Can you work these out from the model? Positions are in its coordinate system, mm. Round coordinates to 2 decimals unless told otherwise and drop trailing zeros. Order: outer loops, then holes, each group sorted by start corner. A loop starts at its lowest first (then second) coordinate and runs counter-clockwise, first axis right, second up.
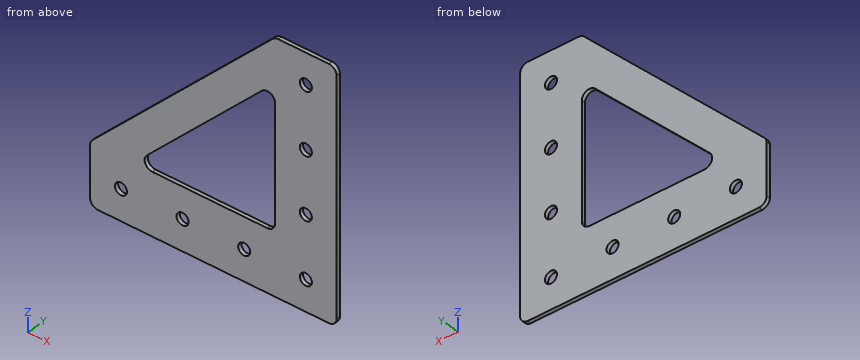
from build123d import *

# Parameters (mm, degrees)
BOSS_EXTRUDE1_DEPTH = 1.5875
SKETCH2_R           = 2.4892
CUT_EXTRUDE1_DEPTH  = 2.5875
LPATTERN1_COUNT     = 4
LPATTERN1_PITCH     = 25.4
LPATTERN1_COL_COUNT = 4
LPATTERN1_COL_PITCH = 25.4
FILLET1_R           = 3.175


with BuildPart() as part:
    # Sketch1 → Boss-Extrude1 (new body)
    with BuildSketch(Plane(origin=(0, 0, 0), x_dir=(1, 0, 0), z_dir=(0, 1, 0))):
        Polygon((0, 0), (-101.6, 0), (-101.6, -25.4), (-25.4, -101.6), (0, -101.6), align=None)
        Polygon((-25.4, -25.4), (-25.4, -83.639487758), (-83.639487758, -25.4), align=None, mode=Mode.SUBTRACT)
    extrude(amount=BOSS_EXTRUDE1_DEPTH)

    # Sketch2 → Cut-Extrude1 (cut, through all)
    with BuildSketch(Plane(origin=(0, 1.5875, 0), x_dir=(1, 0, 0), z_dir=(0, 1, 0))):
        with Locations((-12.7, -12.7)):
            Circle(SKETCH2_R)
    cut_extrude1 = extrude(amount=-CUT_EXTRUDE1_DEPTH, mode=Mode.SUBTRACT)

    # LPattern1: Cut-Extrude1 ×4
    with Locations(*[(0, 0, i * LPATTERN1_PITCH) for i in range(1, LPATTERN1_COUNT)]):
        add(cut_extrude1, mode=Mode.SUBTRACT)

    # LPattern1 col: Cut-Extrude1 ×4
    with Locations(*[(-i * LPATTERN1_COL_PITCH, 0, 0) for i in range(1, LPATTERN1_COL_COUNT)]):
        add(cut_extrude1, mode=Mode.SUBTRACT)

    # Fillet1
    fillet1_edges = [part.edges().sort_by_distance(p)[0] for p in [
        (-83.639487758, 0.79375, 25.4),
        (-25.4, 0.79375, 83.639487758),
        (-25.4, 0.79375, 25.4),
        (0, 0.79375, 101.6),
        (-25.4, 0.79375, 101.6),
        (-101.6, 0.79375, 25.4),
        (-101.6, 0.79375, 0),
        (0, 0.79375, 0),
    ]]
    fillet(fillet1_edges, radius=FILLET1_R)


solid = part.part
(1) I want a section at A-A, the plane z = 88.9. List the corners of the cut face in (x, y) for me.
(2) I want a section at C-C, the plane y = 0.7. Give the number of separate pieces and of enclosed holes in the cut face, plus the area to 3 significant figures.
(3) Please list where these lines run through material, in increasing order: probe 1 along X at (y, z) = (0.3, 12.7); probe 2 along Z at (x, y) = (-12.7, 0.55); probe 3 along X at (y, z) = (0.85, 38).
(4) I want a section at D-D, the plane x = -38.1. List the corners of the cut face in (y, z) for me.
(5) I want a section at B-B, the plane x = -12. List the corners of the cut face in (y, z) for me, plus the area to 3 significant figures.
(6) I'm going to push flat-ended pins straight in: pin 1 Ø4.5 at (x, z) = (-38.1, 12.7) entering from +Y; pin 2 Ø0.5 at (x, y) = (-48.5, 0.5) entering from +Z. Where does each tip first touch, or does it pass through?
Ans:
1. outline: (-38.1, 0) - (-15.19, 0) - (-15.19, 1.59) - (-38.1, 1.59) - close; (-10.21, 0) - (0, 0) - (0, 1.59) - (-10.21, 1.59) - close
2. separate pieces: 1
2. enclosed holes: 8
2. area: 5,610 mm2
3. probe 1: x = -101.6 to -91.39, -86.41 to -65.99, -61.01 to -40.59, -35.61 to -15.19, -10.21 to 0
3. probe 2: z = 0 to 10.21, 15.19 to 35.61, 40.59 to 61.01, 65.99 to 86.41, 91.39 to 101.6
3. probe 3: x = -89 to -71.04, -25.4 to -15.19, -10.21 to 0
4. outline: (0, 0) - (1.59, 0) - (1.59, 10.21) - (0, 10.21) - close; (0, 15.19) - (1.59, 15.19) - (1.59, 25.4) - (0, 25.4) - close; (0, 70.94) - (1.59, 70.94) - (1.59, 88.9) - (0, 88.9) - close
5. outline: (0, 0) - (1.59, 0) - (1.59, 10.31) - (0, 10.31) - close; (0, 15.09) - (1.59, 15.09) - (1.59, 35.71) - (0, 35.71) - close; (0, 40.49) - (1.59, 40.49) - (1.59, 61.11) - (0, 61.11) - close; (0, 65.89) - (1.59, 65.89) - (1.59, 86.51) - (0, 86.51) - close; (0, 91.29) - (1.59, 91.29) - (1.59, 101.6) - (0, 101.6) - close
5. area: 131 mm2
6. pin 1: passes through
6. pin 2: stops at z = 78.75
